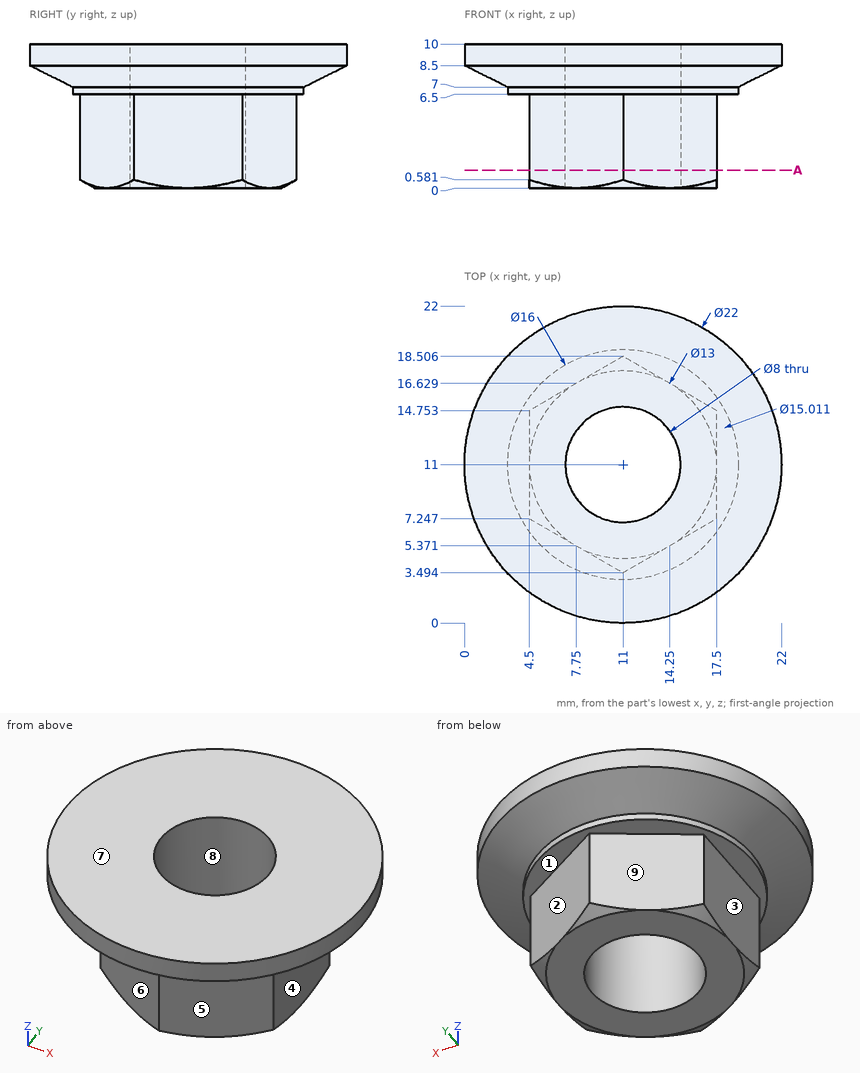
Source: three-view drawing plus pictorial views. Frame: mm from the lowest corner of the part. A direction names the side the tool comes from. Round coordinates to 2 decimals unless told otherwise and drop trailing zeros. Write each loop counter-clockwise with the first axis right and the second up, starting at its lowest first coordinate (ties: lowest second). Pieces come first, ordered by that corner, then holes. Notation, with made-up numbers: (31.5, -22) -> (69.5, -22) arc R26 cw to (69.5, 8) -> close; hole circle Ø3 at (-15, -30). An arc over 180 degrees is marked (long way). Return JSON: item names as keys, results as strings.
Q1. First-contact query: pin 1 Ø2 at (x, z) = (17, 2.5) entering from +Y; pin 2 Ø3 at (y, z) = (13, 5.5) entering from +X; pin 3 Ø1.5 at (y, z) = (9.5, 1.5) entering from +X. Flat tips, straight axial feed; report the tip coordinate or a pass-through.
From the geometry:
{"pin 1": "y = 15.62", "pin 2": "x = 18.95", "pin 3": "x = 17.5"}
Q2. Mould query, pull axis Y, two halves, no side actions, for the marked faces 6, 7, 8 and 9. Classes: +Y half, -Y half, draft (parallel to the pull), parting line (faces both ways), or undercut.
From the geometry:
{"face 6": "-Y half", "face 7": "draft", "face 8": "undercut", "face 9": "+Y half"}
Q3. Ray query, line 1 (Z direction, x = 7.25, y = 5.5); line 2 (X direction, y = 12.5, z = 5); line 3 (X direction, y = 11.5, z = 8) (1 decimal). Return the intervals inside material, ascending.
From the geometry:
{"line 1": "6.5 to 10", "line 2": "4.5 to 7.29, 14.71 to 17.5", "line 3": "1 to 7, 15 to 21"}
Q4. Section A-A on z = 1.25. Return the cut outline in (x, y) (1 decimal).
From the geometry:
{"outline": "(4.5, 7.2) -> (11, 3.5) -> (17.5, 7.2) -> (17.5, 14.8) -> (11, 18.5) -> (4.5, 14.8) -> close; hole circle Ø8 at (11, 11)"}
Q5. Set-up query: the marked faces 1, 2, 3, 4 and 5. Return all of +Z, -Z, +X, -X, +Y, -Y with unobstructed straight access to the full face (end or side cutting, diameter ignored); none if empty.
From the geometry:
{"face 1": "-Z", "face 2": "-Z, +X, +Y", "face 3": "-Z, -X, +Y, -Y", "face 4": "-Z, +X, +Y, -Y", "face 5": "-Z, +X, -Y"}
